Could you check a few things on this model? Use its own coordinates, in mm. A direction names the side the tool comes from. Give positions to 0.01 mm unless a question says otherwise; leave off trailing zeros. Write each loop counter-clockwise with the first axis right and the second up, starting at its lowest first coordinate (ties: lowest second). Pieces come first, ordered by that corner, then holes. Notation, with made-up numbers: (-26.75, -12) -> (30.25, -12) arc R29 cw to (30.25, 14) -> close; hole circle Ø9 at (-26.5, 37.5). An arc over 180 degrees is marked (long way). Write item = value, one per line. Start each with the question number.
```python
from build123d import *

# Parameters (mm, degrees)
BOSS_EXTRUDE1_DEPTH = 8
SKETCH2_R           = 1.5
CUT_EXTRUDE1_DEPTH  = 11.066445914
SKETCH3_R           = 3
CUT_EXTRUDE2_DEPTH  = 6


with BuildPart() as part:
    # Sketch1 → Boss-Extrude1 (new body)
    with BuildSketch(Plane.XY):
        Polygon((-2.309401077, 4), (-4.618802154, 0), (-2.309401077, -4), (2.309401077, -4), (4.618802154, 0), (2.309401077, 4), align=None)
    extrude(amount=BOSS_EXTRUDE1_DEPTH)

    # Sketch2 → Cut-Extrude1 (cut, through all)
    with BuildSketch(Plane.XY.offset(8)):
        Circle(SKETCH2_R)
    extrude(amount=-CUT_EXTRUDE1_DEPTH, mode=Mode.SUBTRACT)

    # Sketch3 → Cut-Extrude2 (cut)
    with BuildSketch(Plane.XY.offset(8)):
        Circle(SKETCH3_R)
    extrude(amount=-CUT_EXTRUDE2_DEPTH, mode=Mode.SUBTRACT)


solid = part.part
```
(1) Imagine slicing it at A-A (x = 0). Please give me the cut outline in (y, z), then the cut area to 3 significant figures.
(2) Imagine slicing it at D-D (z = 0.5). Please give me the cut outline in (x, y).
(3) If I drill on line 1 along Y through (x, z) = (0, 1.05); line 2 along Y through (x, z) = (0, 6.7); line 3 along Z through (x, y) = (2, 2), over which ranges is the centre line in solid material (lowest first)? Write a range as from..to.
(4) We'd pull the mould along X, two halves only. Please class faces 3 (the flat face through (3.448, -2.028, 3.944)), 4 (the flat face through (2, 0, 0)), 5 (the cylindrical face through (-3, 0, 5)): released by +X, released by -X, zero draft, split by the parting line, or undercut.
(5) On a 3-axis mill with a long thin cutter (end or side, diameter ignored), from which of +Z, -Z, +X, -X, +Y, -Y can I reach the whole of each face in a straight line? I mean faces 1 (the flat face through (-3.48, -1.97, 3.94)), 2 (the flat face through (1.3, -1.3, 2)). Say none if no direction works.
(6) I'm going to push flat-ended pins straight in: pin 1 (1 mm diameter, centred on y = 1.5, z = 1, fed in from -X); pin 2 (1.8 mm diameter, centred on x = 0.5, y = -1.5, fed in from +Z). Where does each tip first touch, or does it pass through?
(7) Imagine slicing it at C-C (y = -0.75). Please give me the cut outline in (x, z).
(8) Imagine slicing it at B-B (z = 6.75). Please give me the cut outline in (x, y), then the cut area to 3 significant figures.
Answers below:
q1.outline = (-4, 0) -> (-1.5, 0) -> (-1.5, 2) -> (-3, 2) -> (-3, 8) -> (-4, 8) -> close; (1.5, 0) -> (4, 0) -> (4, 8) -> (3, 8) -> (3, 2) -> (1.5, 2) -> close
q1.area = 22.0 mm^2
q2.outline = (-4.62, 0) -> (-2.31, -4) -> (2.31, -4) -> (4.62, 0) -> (2.31, 4) -> (-2.31, 4) -> close; hole circle Ø3 at (0, 0)
q3.line_1 = -4..-1.5, 1.5..4
q3.line_2 = -4..-3, 3..4
q3.line_3 = 0..2
q4.face_3 = released by +X
q4.face_4 = zero draft
q4.face_5 = undercut
q5.face_1 = +Z, -Z, -X, -Y
q5.face_2 = +Z
q6.pin_1 = -4.04
q6.pin_2 = 2
q7.outline = (-4.19, 0) -> (-1.3, 0) -> (-1.3, 2) -> (-2.9, 2) -> (-2.9, 8) -> (-4.19, 8) -> close; (1.3, 0) -> (4.19, 0) -> (4.19, 8) -> (2.9, 8) -> (2.9, 2) -> (1.3, 2) -> close
q8.outline = (-4.62, 0) -> (-2.31, -4) -> (2.31, -4) -> (4.62, 0) -> (2.31, 4) -> (-2.31, 4) -> close; hole circle Ø6 at (0, 0)
q8.area = 27.2 mm^2
